```python
from build123d import *

# Parameters (mm, degrees)
CROQUIS1_R                 = 30.5
SALIENTE_EXTRUIR1_DEPTH    = 3
CROQUIS2_R                 = 2
CORTAR_EXTRUIR1_DEPTH      = 4
CORTAR_EXTRUIR3_START      = -4
CORTAR_EXTRUIR3_DEPTH      = 4
CORTAR_EXTRUIR5_START      = -4
CORTAR_EXTRUIR5_DEPTH      = 4
CORTAR_EXTRUIR6_DEPTH      = 10
CROQUIS10_R                = 2.5
CORTAR_EXTRUIR7_DEPTH      = 3
CORTAR_EXTRUIR8_DEPTH      = 44.237715166
CORTAR_EXTRUIR8_DEPTH_BACK = 44.237715166


with BuildPart() as part:
    # Croquis1 → Saliente-Extruir1 (new body)
    with BuildSketch(Plane(origin=(0, 0, 0), x_dir=(1, 0, 0), z_dir=(0, 1, 0))):
        with Locations(Location((0, 0, 0), (0, 0, 270))):
            Circle(CROQUIS1_R)
    extrude(amount=SALIENTE_EXTRUIR1_DEPTH)

    # Croquis2 → Cortar-Extruir1 (cut)
    with BuildSketch(Plane(origin=(0, 3, 0), x_dir=(1, 0, 0), z_dir=(0, 1, 0))):
        with Locations(Location((0, 0, 0), (0, 0, 270))):
            Circle(CROQUIS2_R)
    extrude(amount=-CORTAR_EXTRUIR1_DEPTH, mode=Mode.SUBTRACT)

    # Croquis5 → Cortar-Extruir3 (cut)
    with BuildSketch(Plane(origin=(0, 3, 0), x_dir=(1, 0, 0), z_dir=(0, 1, 0)).offset(CORTAR_EXTRUIR3_START)):
        with BuildLine():
            Line((28.814059068, 5), (30.087372767, 5))
            ThreePointArc((30.087372767, 5), (29.556634924, 7.526973624), (28.814059068, 10))
            Line((28.814059068, 10), (24.814059068, 10))
            Line((24.814059068, 10), (24.814059068, 5))
            Line((24.814059068, 5), (28.814059068, 5))
        make_face()
        with BuildLine():
            Line((30.087372767, -5), (28.814059068, -5))
            Line((28.814059068, -5), (24.814059068, -5))
            Line((24.814059068, -5), (24.814059068, -10))
            Line((24.814059068, -10), (28.814059068, -10))
            ThreePointArc((28.814059068, -10), (29.556634924, -7.526973624), (30.087372767, -5))
        make_face()
        with BuildLine():
            Line((-24.814059068, 5), (-24.814059068, 10))
            Line((-24.814059068, 10), (-28.814059068, 10))
            ThreePointArc((-28.814059068, 10), (-29.556634924, 7.526973624), (-30.087372767, 5))
            Line((-30.087372767, 5), (-28.814059068, 5))
            Line((-28.814059068, 5), (-24.814059068, 5))
        make_face()
        with BuildLine():
            Line((-28.814059068, -10), (-24.814059068, -10))
            Line((-24.814059068, -10), (-24.814059068, -5))
            Line((-24.814059068, -5), (-28.814059068, -5))
            Line((-28.814059068, -5), (-30.087372767, -5))
            ThreePointArc((-30.087372767, -5), (-29.556634924, -7.526973624), (-28.814059068, -10))
        make_face()
    extrude(amount=CORTAR_EXTRUIR3_DEPTH, mode=Mode.SUBTRACT)

    # Croquis7 → Cortar-Extruir5 (cut)
    with BuildSketch(Plane(origin=(0, 3, 0), x_dir=(1, 0, 0), z_dir=(0, 1, 0)).offset(CORTAR_EXTRUIR5_START)):
        Polygon((1.428390211, 22.411430151), (-0.869743118, 20.483067322), (2.34419493, 16.652845106), (4.642328259, 18.581207935), align=None)
        with BuildLine():
            Line((-24.814059068, -10), (-28.814059068, -10))
            ThreePointArc((-28.814059068, -10), (0, -30.5), (28.814059068, -10))
            Line((28.814059068, -10), (24.814059068, -10))
            add(Edge.make_bspline(
                [(24.814059068, -10), (22.863263717, -9.657344338), (20.984021298, -8.980450277), (19.168992989, -8.065339906)],
                knots=[0, 0, 0, 0, 0.087850084, 0.087850084, 0.087850084, 0.087850084], degree=3))
            Line((19.168992989, -8.065339906), (11.455541673, 1.127193412))
            Line((11.455541673, 1.127193412), (9.248678515, -0.72458465))
            add(Edge.make_bspline(
                [(9.248678515, -0.72458465), (4.033234859, 4.116641048), (-0.646914404, 9.508508747), (-5.04935939, 12.080675515)],
                knots=[0.258799312, 0.258799312, 0.258799312, 0.258799312, 0.546435258, 0.546435258, 0.546435258, 0.546435258], degree=3))
            Line((-5.04935939, 12.080675515), (-0.757422911, 15.682037831))
            Line((-0.757422911, 15.682037831), (-7.828086618, 24.108526705))
            Line((-7.828086618, 24.108526705), (-17.020619935, 16.395075389))
            Line((-17.020619935, 16.395075389), (-13.66601447, 12.397212273))
            add(Edge.make_bspline(
                [(-13.66601447, 12.397212273), (-17.403465693, 9.897923685), (-21.056529869, 3.255841362), (-24.814059068, -10)],
                knots=[0.740637404, 0.740637404, 0.740637404, 0.740637404, 1, 1, 1, 1], degree=3))
        make_face()
        Polygon((14.685884661, 6.611763511), (12.387751331, 4.683400682), (15.60168938, 0.853178467), (17.899822709, 2.781541296), align=None)
    extrude(amount=CORTAR_EXTRUIR5_DEPTH, mode=Mode.SUBTRACT)

    # Croquis9 → Cortar-Extruir6 (cut)
    with BuildSketch(Plane(origin=(0, 3, 0), x_dir=(1, 0, 0), z_dir=(0, 1, 0))):
        Polygon((7.971418181, 14.613753061), (5.673284852, 12.685390231), (8.887222901, 8.855168016), (11.18535623, 10.783530845), align=None)
    extrude(amount=-CORTAR_EXTRUIR6_DEPTH, mode=Mode.SUBTRACT)

    # Croquis10 → Cortar-Extruir7 (cut)
    with BuildSketch(Plane(origin=(0, 3, 0), x_dir=(1, 0, 0), z_dir=(0, 1, 0))):
        with Locations(Location((12, 16, 0), (0, 0, 270))):
            Circle(CROQUIS10_R)
    extrude(amount=-CORTAR_EXTRUIR7_DEPTH, mode=Mode.SUBTRACT)

    # Croquis11 → Cortar-Extruir8 (cut, two sides: drawn at the far end of the back side and taken through both)
    with BuildSketch(Plane(origin=(0, 3, 0), x_dir=(1, 0, 0), z_dir=(0, 1, 0)).offset(-CORTAR_EXTRUIR8_DEPTH_BACK)):
        with BuildLine():
            Line((30.087372767, 5), (27.814059068, 5))
            Line((27.814059068, 5), (27.814059068, -5))
            Line((27.814059068, -5), (30.087372767, -5))
            ThreePointArc((30.087372767, -5), (30.5, 0), (30.087372767, 5))
        make_face()
        with BuildLine():
            ThreePointArc((28.814059068, 10), (28.341972277, 11.268655974), (27.814059068, 12.515115586))
            Line((27.814059068, 12.515115586), (27.814059068, 10))
            Line((27.814059068, 10), (28.814059068, 10))
        make_face()
        with BuildLine():
            Line((-27.814059068, -5), (-27.814059068, 5))
            Line((-27.814059068, 5), (-30.087372767, 5))
            ThreePointArc((-30.087372767, 5), (-30.5, 0), (-30.087372767, -5))
            Line((-30.087372767, -5), (-27.814059068, -5))
        make_face()
        with BuildLine():
            Line((-28.814059068, 10), (-27.814059068, 10))
            Line((-27.814059068, 10), (-27.814059068, 12.515115586))
            ThreePointArc((-27.814059068, 12.515115586), (-28.341972277, 11.268655974), (-28.814059068, 10))
        make_face()
    extrude(amount=CORTAR_EXTRUIR8_DEPTH + CORTAR_EXTRUIR8_DEPTH_BACK, mode=Mode.SUBTRACT)


solid = part.part
```
Part model, mm, in its own coordinate system. A direction names the side the tool comes from. Give positions to 0.01 mm unless a question says otherwise; leave off trailing zeros. Loops run counter-clockwise (first coordinate to the right, second up) from the corner with the lowest first, then second, coordinate; pieces in that order, holes last. Notation, with made-up numbers: M 44,20.5 L 103,20.5 A11 cw 103,25.5 Z; hole C 47,16 d6. An arc over 180 degrees is marked long. Return JSON: item names as keys, results as strings.
1) Pull direction Z, two halves, no side cores. Call faces 1 (the face through (-15.367, 1.479, -14.424)), 2 (the face through (15.366, 1.479, 3.533)), 3 (the face through (24.814, 1, 7)): released by +Z, released by -Z, zero draft, split by the parting line, or undercut.
Calculated:
{"face 1": "undercut", "face 2": "released by +Z", "face 3": "zero draft"}
2) Drill centre lines: line 1 (X direction, y = 1.95, z = -14.5); line 2 (X direction, y = 1.8, z = -16); line 3 (X direction, y = 2.4, z = -15). Where is each one in solid material? Low to high.
Calculated:
{"line 1": "x = -26.83 to -15.43, -2.17 to 7.84, 8.07 to 10, 14 to 26.83", "line 2": "x = -25.97 to -16.69, -1.02 to 9.5, 14.5 to 25.97", "line 3": "x = -26.56 to -15.85, -1.57 to 9.71, 14.29 to 26.56"}
3) 3-axis set-ups, long thin cutter, end or side, ignore diameter. For faces 4 (the face through (26, 1, -10)), 5 (the face through (7.258, 1.521, -10.797)), 6 (the face through (-24.814, 1, 8)), 7 (the face through (-26, 1, -5)), 8 (the face through (10.368, 1.479, -0.214)): which of +Z, -Z, +X, -X, +Y, -Y reach the whole face in a straight line?
Calculated:
{"face 4": "+X, +Y, -Y", "face 5": "+Y, -Y", "face 6": "+Z, -X, +Y, -Y", "face 7": "-X, +Y, -Y", "face 8": "+Z, +Y, -Y"}
4) Flat gauge pins, fed straight in: pin 1 Ø1.5 at (y, z) = (1.5, -20) entering from +X; pin 2 Ø1.5 at (x, y) = (-27, 2) entering from +Z; pin 3 Ø0.9 at (y, z) = (1.5, -6.5) entering from +X. Where does each tip first touch, or does it go through?
Calculated:
{"pin 1": "stops at x = 23.66", "pin 2": "stops at z = 5", "pin 3": "stops at x = 24.81"}
5) Saw through at B-B, the plane x = -12. List the corners of the cut face in (y, z), then the cut area to 3 significant figures.
Calculated:
{"outline": "M 0,-28.04 L 3,-28.04 L 3,-20.61 L 0,-20.61 Z", "area": "22.3 mm2"}
6) Saw through at A-A, the plane y = 1.9. Count the separate pieces of the cut face and the enclosed holes in it, then the cut area to 3 significant figures.
Calculated:
{"separate pieces": "1", "enclosed holes": "4", "area": "1,080 mm2"}
